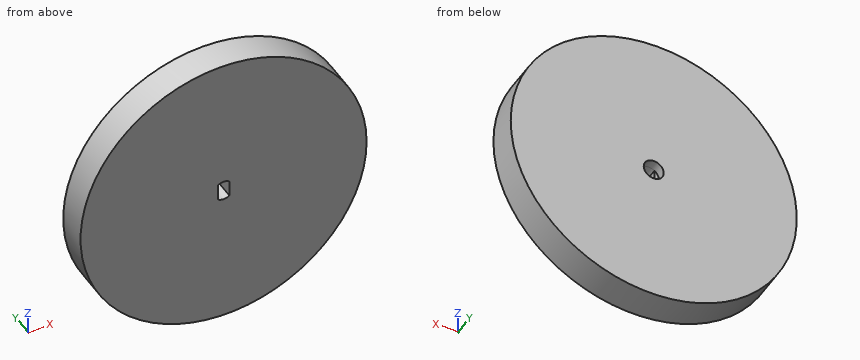
from build123d import *

# Parameters (mm, degrees)
SKETCH1_R           = 37.5
BOSS_EXTRUDE1_DEPTH = 8.5
SKETCH2_R           = 2.625
CUT_EXTRUDE1_DEPTH  = 2.5
CUT_EXTRUDE2_DEPTH  = 6


with BuildPart() as part:
    # Sketch1 → Boss-Extrude1 (new body)
    with BuildSketch(Plane(origin=(0, 0, 0), x_dir=(1, 0, 0), z_dir=(0, 1, 0))):
        Circle(SKETCH1_R)
    extrude(amount=BOSS_EXTRUDE1_DEPTH)

    # Sketch2 → Cut-Extrude1 (cut)
    with BuildSketch(Plane(origin=(0, 8.5, 0), x_dir=(1, 0, 0), z_dir=(0, 1, 0))):
        Circle(SKETCH2_R)
    extrude(amount=-CUT_EXTRUDE1_DEPTH, mode=Mode.SUBTRACT)

    # Sketch3 → Cut-Extrude2 (cut)
    with BuildSketch(Plane(origin=(0, 6, 0), x_dir=(1, 0, 0), z_dir=(0, 1, 0))):
        with BuildLine():
            Line((-1.525, 2.136586062), (-1.525, -2.136586062))
            ThreePointArc((-1.525, -2.136586062), (0, -2.625), (1.525, -2.136586062))
            Line((1.525, -2.136586062), (1.525, 2.136586062))
            ThreePointArc((1.525, 2.136586062), (0, 2.625), (-1.525, 2.136586062))
        make_face()
    extrude(amount=-CUT_EXTRUDE2_DEPTH, mode=Mode.SUBTRACT)


solid = part.part
Read the model definition and answer for the solid it produces. Units are mm, in the model's axes. Coordinates: 2 decimals unless noted, no trailing zeros. Order: outer loops, then holes, each group sorted by start corner. A loop starts at its lowest first (then second) coordinate and runs counter-clockwise, first axis right, second up. Notation, with made-up numbers: M 28,-9.5 L 81,-9.5 A24 ccw 81,12.5 Z; hole C 32,80 d5. An arc over 180 degrees is marked long. Put each result on its own line as item: value. Start each with the question number.
Item 1: Section A-A, the plane z = 0 is taken. Determine the outline of the cut face in (x, y) (3 decimals), plus the area to 3 significant figures.
Item 2: Section C-C, the plane x = 0 is taken. Determine the outline of the cut face in (y, z) (3 decimals), plus the area to 3 significant figures.
Item 3: Given pin 1 Ø0.6 at (x, z) = (2, 0) entering from +Y; pin 2 Ø5 at (x, y) = (-3, 5) entering from -Z; pin 3 Ø5 at (x, y) = (-13.5, 7.5) entering from -Z, each flat-ended and moving along its own axis, determine where each tip first touches the part or whether it passes through.
Item 4: Section D-D, the plane z = -21 is taken. Determine the outline of the cut face in (x, y), plus the area to 3 significant figures.
Item 5: Section B-B, the plane y = 4.5 is taken. Determine the outline of the cut face in (x, z) (3 decimals), plus the area to 3 significant figures.
Item 6: Consider probe 1 along Z at (x, y) = (0, 7.4) (3 decimals); probe 2 along X at (y, z) = (6.5, -2). Determine where each line is inside the solid, lowest interval first. Write a range as [from, to].
Computed:
1. outline: M -37.5,0 L -1.525,0 L -1.525,6 L -2.625,6 L -2.625,8.5 L -37.5,8.5 Z; M 1.525,0 L 37.5,0 L 37.5,8.5 L 2.625,8.5 L 2.625,6 L 1.525,6 Z
1. area: 606 mm2
2. outline: M 0,-37.5 L 8.5,-37.5 L 8.5,-2.625 L 0,-2.625 Z; M 0,2.625 L 8.5,2.625 L 8.5,37.5 L 0,37.5 Z
2. area: 593 mm2
3. pin 1: stops at y = 6
3. pin 2: stops at z = -37.5
3. pin 3: stops at z = -35.85
4. outline: M -31.07,0 L 31.07,0 L 31.07,8.5 L -31.07,8.5 Z
4. area: 528 mm2
5. outline: C 0,0 d75; hole M -1.525,-2.137 A2.625 ccw 1.525,-2.137 L 1.525,2.137 A2.625 ccw -1.525,2.137 Z
5. area: 4,400 mm2
6. probe 1: z = [-37.5, -2.625], [2.625, 37.5]
6. probe 2: x = [-37.45, -1.7], [1.7, 37.45]
